Build history of the part. All positions in model axes, mm. Face numbers are marked on the shaded views. A direction names the side the tool comes from. Give positions to 0.01 mm unless a question says otherwise; leave off trailing zeros. Order: outer loops, then holes, each group sorted by start corner. A loop starts at its lowest first (then second) coordinate and runs counter-clockwise, first axis right, second up. Notation, with made-up numbers: (-34, -4) -> (20, -4) arc R23 ccw to (20, 33) -> close; hole circle Ø6 at (-23.75, 56.25). An arc over 180 degrees is marked (long way). Use a Markdown table: item, result. Add a question column.
```python
from build123d import *

# Parameters (mm, degrees)
F1_DEPTH = 19.05
F2_R     = 2.54


with BuildPart() as f1:
    # F0 (on Top) → F1 (new body)
    with BuildSketch(Plane.XY):
        Polygon((19.05, 38.1), (0, 38.1), (0, 0), (19.05, 0), (19.05, 19.05), (38.1, 19.05), (38.1, 38.1), (57.15, 38.1), (57.15, 57.15), (19.05, 57.15), align=None)
    extrude(amount=F1_DEPTH)

    # F2
    f2_edges = [f1.edges().sort_by_distance(p)[0] for p in [
        (38.1, 57.15, 19.05),
        (19.05, 47.625, 19.05),
        (9.525, 38.1, 19.05),
        (0, 19.05, 19.05),
        (9.525, 0, 19.05),
        (19.05, 9.525, 19.05),
        (28.575, 19.05, 19.05),
        (38.1, 28.575, 19.05),
        (47.625, 38.1, 19.05),
        (57.15, 47.625, 19.05),
        (38.1, 57.15, 0),
        (19.05, 47.625, 0),
        (9.525, 38.1, 0),
        (0, 19.05, 0),
        (9.525, 0, 0),
        (19.05, 9.525, 0),
        (28.575, 19.05, 0),
        (38.1, 28.575, 0),
        (47.625, 38.1, 0),
        (57.15, 47.625, 0),
        (0, 0, 9.525),
        (19.05, 0, 9.525),
        (57.15, 38.1, 9.525),
        (57.15, 57.15, 9.525),
        (38.1, 19.05, 9.525),
        (19.05, 57.15, 9.525),
        (0, 38.1, 9.525),
    ]]
    fillet(f2_edges, radius=F2_R)


solid = f1.part
```
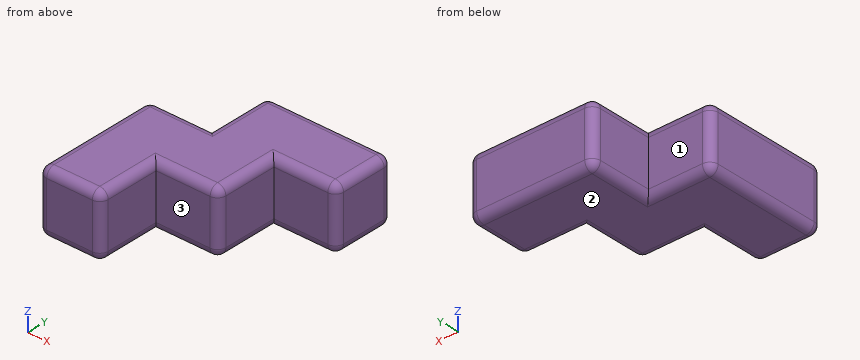
(1) Wall check: probe 1 along Y at (x, z) = (10.5, 3.75); probe 2 along Y at (x, z) = (40.5, 11.25); probe 3 along X at (y, z) = (45.5, 16.25). Give the ranges that are in metal, low to high.
(2) Band-saw the part on A-A on y = 10. Give the cut face in (x, z), plus the area to 3 significant figures.
(3) Band-saw the part on C-C on z = 8.5. Give the cut face in (x, y).
(4) Pin check, flat tips, straight feed: pin 1 Ø11 at (y, z) = (32.5, 8) entering from +X; pin 2 Ø7 at (x, z) = (28.5, 8) entering from -Y; pin 3 Ø11 at (y, z) = (48, 9) entering from -X. Stop position of each tip, or through.
(5) Band-saw the part on B-B on x = 40. Give the cut face in (y, z), plus the area to 3 significant figures.
(6) Tool access for the marked faces 1, 2 and 3: list every direction of +Z, -Z, +X, -X, +Y, -Y with a clear straight run to the whole face (end or side of a thin tool).
Response:
| question | item | result |
|---|---|---|
| 1 | probe 1 | y = 0 to 38.1 |
| 1 | probe 2 | y = 38.1 to 57.15 |
| 1 | probe 3 | x = 19.05 to 57.15 |
| 2 | outline | (0, 2.54) arc R2.54 ccw to (2.54, 0) -> (16.51, 0) arc R2.54 ccw to (19.05, 2.54) -> (19.05, 16.51) arc R2.54 ccw to (16.51, 19.05) -> (2.54, 19.05) arc R2.54 ccw to (0, 16.51) -> close |
| 2 | area | 357 mm² |
| 3 | outline | (0, 2.54) arc R2.54 ccw to (2.54, 0) -> (16.51, 0) arc R2.54 ccw to (19.05, 2.54) -> (19.05, 19.05) -> (35.56, 19.05) arc R2.54 ccw to (38.1, 21.59) -> (38.1, 38.1) -> (54.61, 38.1) arc R2.54 ccw to (57.15, 40.64) -> (57.15, 54.61) arc R2.54 ccw to (54.61, 57.15) -> (21.59, 57.15) arc R2.54 ccw to (19.05, 54.61) -> (19.05, 38.1) -> (2.54, 38.1) arc R2.54 ccw to (0, 35.56) -> close |
| 4 | pin 1 | stops at x = 38.1 |
| 4 | pin 2 | stops at y = 19.05 |
| 4 | pin 3 | stops at x = 19.05 |
| 5 | outline | (38.1, 2.54) arc R2.54 ccw to (40.64, 0) -> (54.61, 0) arc R2.54 ccw to (57.15, 2.54) -> (57.15, 16.51) arc R2.54 ccw to (54.61, 19.05) -> (40.64, 19.05) arc R2.54 ccw to (38.1, 16.51) -> close |
| 5 | area | 357 mm² |
| 6 | face 1 | +Z, -Z, -X, +Y |
| 6 | face 2 | -Z, +X, -X, +Y, -Y |
| 6 | face 3 | +Z, -Z, +X, -Y |
